```python
from build123d import *

# Parameters (mm, degrees)
SKETCH_1_W          = 206.4
SKETCH_1_H          = 150
SKETCH_1_R          = 2.1
SKETCH_1_R_2        = 1.5
EXTRUDE_1_DEPTH     = 3
CUT_EXTRUDE_1_DEPTH = 153.892903694
FILLET_1_R          = 3
CUT_EXTRUDE_2_DEPTH = 2
SKETCH_6_R          = 10
CUT_EXTRUDE_3_DEPTH = 10
SKETCH_7_W          = 45
SKETCH_7_H          = 100
CUT_EXTRUDE_4_DEPTH = 10
FILLET_2_R          = 3
SKETCH_8_W          = 45.884132908
SKETCH_8_H          = 94.377965814
CUT_EXTRUDE_5_DEPTH = 10
SKETCH_9_W          = 66.4
SKETCH_9_H          = 90
CUT_EXTRUDE_6_DEPTH = 10
SKETCH_10_R         = 1.5
CUT_EXTRUDE_7_DEPTH = 2


with BuildPart() as part:
    # 草图1 → 凸台-拉伸1 (new body)
    with BuildSketch(Plane(origin=(0, 0, 0), x_dir=(1, 0, 0), z_dir=(0, 1, 0))):
        with Locations((-30, 0)):
            Rectangle(SKETCH_1_W, SKETCH_1_H)
        with Locations(Location((65.7, 67.5, 0), (0, 0, 270))):
            Circle(SKETCH_1_R, mode=Mode.SUBTRACT)
        with Locations(Location((65.7, -67.5, 0), (0, 0, 90))):
            Circle(SKETCH_1_R, mode=Mode.SUBTRACT)
        with Locations(Location((-65.7, -67.5, 0), (0, 0, 270))):
            Circle(SKETCH_1_R, mode=Mode.SUBTRACT)
        with Locations(Location((-65.7, 67.5, 0), (0, 0, 90))):
            Circle(SKETCH_1_R, mode=Mode.SUBTRACT)
        with Locations(Location((-65.7, 37.5, 0), (0, 0, 270))):
            Circle(SKETCH_1_R, mode=Mode.SUBTRACT)
        with Locations(Location((-40.7, 37.5, 0), (0, 0, 270))):
            Circle(SKETCH_1_R, mode=Mode.SUBTRACT)
        with Locations(Location((-40.7, 67.5, 0), (0, 0, 270))):
            Circle(SKETCH_1_R, mode=Mode.SUBTRACT)
        with Locations(Location((-40.7, -67.5, 0), (0, 0, 270))):
            Circle(SKETCH_1_R, mode=Mode.SUBTRACT)
        with Locations(Location((-40.7, -37.5, 0), (0, 0, 270))):
            Circle(SKETCH_1_R, mode=Mode.SUBTRACT)
        with Locations(Location((-65.7, -37.5, 0), (0, 0, 270))):
            Circle(SKETCH_1_R, mode=Mode.SUBTRACT)
        with Locations(Location((40.7, -67.5, 0), (0, 0, 270))):
            Circle(SKETCH_1_R, mode=Mode.SUBTRACT)
        with Locations(Location((40.7, -37.5, 0), (0, 0, 270))):
            Circle(SKETCH_1_R, mode=Mode.SUBTRACT)
        with Locations(Location((65.7, -37.5, 0), (0, 0, 270))):
            Circle(SKETCH_1_R, mode=Mode.SUBTRACT)
        with Locations(Location((65.7, 37.5, 0), (0, 0, 270))):
            Circle(SKETCH_1_R, mode=Mode.SUBTRACT)
        with Locations(Location((40.7, 37.5, 0), (0, 0, 270))):
            Circle(SKETCH_1_R, mode=Mode.SUBTRACT)
        with Locations(Location((40.7, 67.5, 0), (0, 0, 270))):
            Circle(SKETCH_1_R, mode=Mode.SUBTRACT)
        with Locations(Location((-98.4, 63.575, 0), (0, 0, 270))):
            Circle(SKETCH_1_R_2, mode=Mode.SUBTRACT)
        with Locations(Location((-88.4, 63.575, 0), (0, 0, 270))):
            Circle(SKETCH_1_R_2, mode=Mode.SUBTRACT)
        with Locations(Location((-111.4, 63.575, 0), (0, 0, 270))):
            Circle(SKETCH_1_R_2, mode=Mode.SUBTRACT)
        with Locations(Location((-121.4, 63.575, 0), (0, 0, 270))):
            Circle(SKETCH_1_R_2, mode=Mode.SUBTRACT)
        with Locations(Location((-121.4, -63.474999999, 0), (0, 0, 270))):
            Circle(SKETCH_1_R_2, mode=Mode.SUBTRACT)
        with Locations(Location((-111.4, -63.474999999, 0), (0, 0, 270))):
            Circle(SKETCH_1_R_2, mode=Mode.SUBTRACT)
        with Locations(Location((-98.4, -63.425, 0), (0, 0, 270))):
            Circle(SKETCH_1_R_2, mode=Mode.SUBTRACT)
        with Locations(Location((-88.4, -63.425, 0), (0, 0, 270))):
            Circle(SKETCH_1_R_2, mode=Mode.SUBTRACT)
    extrude(amount=EXTRUDE_1_DEPTH)

    # 草图2 → 切除-拉伸1 (cut, through all)
    with BuildSketch(Plane(origin=(0, 0, 0), x_dir=(1, 0, 0), z_dir=(0, 1, 0))):
        with BuildLine():
            Line((-125.2, -66.425), (-116.5, -66.425))
            ThreePointArc((-116.5, -66.425), (-114.9, -64.825), (-113.3, -66.425))
            Line((-113.3, -66.425), (-113.3, -69.575))
            ThreePointArc((-113.3, -69.575), (-114.9, -71.175), (-116.5, -69.575))
            Line((-116.5, -69.575), (-125.2, -69.575))
            ThreePointArc((-125.2, -69.575), (-126.8, -71.175), (-128.4, -69.575))
            Line((-128.4, -69.575), (-128.4, -66.425))
            ThreePointArc((-128.4, -66.425), (-126.8, -64.825), (-125.2, -66.425))
        make_face()
        with BuildLine():
            Line((-85.2, -66.425), (-76.5, -66.425))
            ThreePointArc((-76.5, -66.425), (-74.9, -64.825), (-73.3, -66.425))
            Line((-73.3, -66.425), (-73.3, -69.575))
            ThreePointArc((-73.3, -69.575), (-74.9, -71.175), (-76.5, -69.575))
            Line((-76.5, -69.575), (-85.2, -69.575))
            ThreePointArc((-85.2, -69.575), (-86.8, -71.175), (-88.4, -69.575))
            Line((-88.4, -69.575), (-88.4, -66.425))
            ThreePointArc((-88.4, -66.425), (-86.8, -64.825), (-85.2, -66.425))
        make_face()
        with BuildLine():
            Line((-73.3, 66.425), (-73.3, 69.575))
            ThreePointArc((-73.3, 69.575), (-74.9, 71.175), (-76.5, 69.575))
            Line((-76.5, 69.575), (-85.2, 69.575))
            ThreePointArc((-85.2, 69.575), (-86.8, 71.175), (-88.4, 69.575))
            Line((-88.4, 69.575), (-88.4, 66.425))
            ThreePointArc((-88.4, 66.425), (-86.8, 64.825), (-85.2, 66.425))
            Line((-85.2, 66.425), (-76.5, 66.425))
            ThreePointArc((-76.5, 66.425), (-74.9, 64.825), (-73.3, 66.425))
        make_face()
        with BuildLine():
            Line((-113.3, 66.425), (-113.3, 69.575))
            ThreePointArc((-113.3, 69.575), (-114.9, 71.175), (-116.5, 69.575))
            Line((-116.5, 69.575), (-125.2, 69.575))
            ThreePointArc((-125.2, 69.575), (-126.8, 71.175), (-128.4, 69.575))
            Line((-128.4, 69.575), (-128.4, 66.425))
            ThreePointArc((-128.4, 66.425), (-126.8, 64.825), (-125.2, 66.425))
            Line((-125.2, 66.425), (-116.5, 66.425))
            ThreePointArc((-116.5, 66.425), (-114.9, 64.825), (-113.3, 66.425))
        make_face()
    extrude(amount=CUT_EXTRUDE_1_DEPTH, mode=Mode.SUBTRACT)

    # 圆角1
    fillet_1_edges = [part.edges().sort_by_distance(p)[0] for p in [
        (73.2, 1.5, 75),
        (-133.2, 1.5, 75),
        (-133.2, 1.5, -75),
        (73.2, 1.5, -75),
    ]]
    fillet(fillet_1_edges, radius=FILLET_1_R)

    # 草图4 → 切除-拉伸2 (cut)
    with BuildSketch(Plane(origin=(0, 0, 0), x_dir=(1, 0, 0), z_dir=(0, 1, 0))):
        with BuildLine():
            Line((-120.7, -27.5), (60.7, -27.5))
            ThreePointArc((60.7, -27.5), (64.235533906, -26.035533906), (65.7, -22.5))
            Line((65.7, -22.5), (65.7, 22.5))
            ThreePointArc((65.7, 22.5), (64.235533906, 26.035533906), (60.7, 27.5))
            Line((60.7, 27.5), (-120.7, 27.5))
            ThreePointArc((-120.7, 27.5), (-124.235533906, 26.035533906), (-125.7, 22.5))
            Line((-125.7, 22.5), (-125.7, -22.5))
            ThreePointArc((-125.7, -22.5), (-124.235533906, -26.035533906), (-120.7, -27.5))
        make_face()
    extrude(amount=CUT_EXTRUDE_2_DEPTH, mode=Mode.SUBTRACT)

    # 草图6 → 切除-拉伸3 (cut)
    with BuildSketch(Plane(origin=(0, 3, 0), x_dir=(1, 0, 0), z_dir=(0, 1, 0))):
        with Locations(Location((0, 0, 0), (0, 0, 270))):
            Circle(SKETCH_6_R)
    extrude(amount=-CUT_EXTRUDE_3_DEPTH, mode=Mode.SUBTRACT)

    # 草图7 → 切除-拉伸4 (cut)
    with BuildSketch(Plane(origin=(0, 3, 0), x_dir=(1, 0, 0), z_dir=(0, 1, 0))):
        with Locations((-110.7, 0)):
            Rectangle(SKETCH_7_W, SKETCH_7_H)
    extrude(amount=-CUT_EXTRUDE_4_DEPTH, mode=Mode.SUBTRACT)

    # 圆角2
    fillet_2_edges = [part.edges().sort_by_distance(p)[0] for p in [
        (-133.2, 1.5, 50),
        (-133.2, 1.5, -50),
        (-88.2, 1.5, -50),
        (-88.2, 1.5, 50),
    ]]
    fillet(fillet_2_edges, radius=FILLET_2_R)

    # 草图8 → 切除-拉伸5 (cut)
    with BuildSketch(Plane(origin=(0, 3, 0), x_dir=(1, 0, 0), z_dir=(0, 1, 0))):
        Rectangle(SKETCH_8_W, SKETCH_8_H)
    extrude(amount=-CUT_EXTRUDE_5_DEPTH, mode=Mode.SUBTRACT)

    # 草图9 → 切除-拉伸6 (cut)
    with BuildSketch(Plane(origin=(0, 3, 0), x_dir=(1, 0, 0), z_dir=(0, 1, 0))):
        with Locations((-1e-09, 0)):
            Rectangle(SKETCH_9_W, SKETCH_9_H)
    extrude(amount=-CUT_EXTRUDE_6_DEPTH, mode=Mode.SUBTRACT)

    # 草图10 → 切除-拉伸7 (cut)
    with BuildSketch(Plane(origin=(0, 3, 0), x_dir=(1, 0, 0), z_dir=(0, 1, 0))):
        with Locations(Location((-15, 60.780217665, 0), (0, 0, 270))):
            Circle(SKETCH_10_R)
        with Locations(Location((15, 60.780217665, 0), (0, 0, 90))):
            Circle(SKETCH_10_R)
        with Locations(Location((15, -60.780217665, 0), (0, 0, 270))):
            Circle(SKETCH_10_R)
        with Locations(Location((-15, -60.780217665, 0), (0, 0, 90))):
            Circle(SKETCH_10_R)
    extrude(amount=-CUT_EXTRUDE_7_DEPTH, mode=Mode.SUBTRACT)


solid = part.part
```
Model file for the job. Use its own axes, mm. A direction names the side the tool comes from. Give positions to 0.01 mm unless a question says otherwise; leave off trailing zeros. Loops run counter-clockwise (first coordinate to the right, second up) from the corner with the lowest first, then second, coordinate; pieces in that order, holes last. Notation, with made-up numbers: (73.25, 69.5) - (91.25, 69.5) arc R28 ccw to (91.25, 89.5) - close; hole circle Ø5 at (62, -14.75). An arc over 180 degrees is marked (long way). One line per item, written item: value. Start each with the question number.
1. Probe L1, parallel to X at y = 2, z = 37.5; L2, parallel to X at y = 0.6, z = -63.5; L3, parallel to Z at x = -41, y = 0.9. List the from-to ranges inside material, lowest first. Write a range as from..to.
2. Slice it at C-C (z = -37.5). List the corners of the cut face in (x, y).
3. Slice it at A-A (x = 40.7). List the corners of the cut face in (y, z), plus the area to 3 significant figures.
4. Pin check, flat tips, straight feed: pin 1 (0.9 mm diameter, centred on x = -15.5, z = 61.5, fed in from +Y); pin 2 (16.5 mm diameter, centred on x = -51, z = 11, fed in from -Y). Stop position of each tip, or through.
5. Pull direction X, two halves, no side cores. Call faces 3 (the cylindrical face through (39.422, 1.479, -39.166)), 4 (the cylindrical face through (64.2, 0.99, 26.07)), 5 (the cylindrical face through (63.65, 1.48, -67.96)), 6 (the flat face through (-54, 3, -1)): pulls with the +X half, pulls with the -X half, needs draft (parallel to the pull), parting line crosses it, or undercut.
6. Which spindle directions (+Z, -Z, +X, -X, +Y, -Y) get a long thin tool onto all of the face, cutting with end or side? Do faces 1 (the cylindrical face through (63.65, 1.48, -37.96)), 2 (the flat face through (49, 2, 0)). Say none if no direction does.
7. Slice it at D-D (x = -8). List the corners of the cut face in (y, z), plus the area to 3 significant figures.
8. Slice it at B-B (x = -81). List the corners of the cut face in (y, z) (3 decimals).
Solution:
1. L1: x = -88.2..-67.8, -63.6..-42.8, -38.6..-33.2, 33.2..38.6, 42.8..63.6, 67.8..73.2
1. L2: x = -133.2..-122.9, -119.9..-112.9, -109.9..-99.9, -96.9..-89.9, -86.9..73.2
1. L3: z = -75..-69.58, -65.42..-39.58, -35.42..-27.5, 27.5..35.42, 39.58..65.42, 69.58..75
2. outline: (-88.2, 0) - (-67.8, 0) - (-67.8, 3) - (-88.2, 3) - close; (-63.6, 0) - (-42.8, 0) - (-42.8, 3) - (-63.6, 3) - close; (-38.6, 0) - (-33.2, 0) - (-33.2, 3) - (-38.6, 3) - close; (33.2, 0) - (38.6, 0) - (38.6, 3) - (33.2, 3) - close; (42.8, 0) - (63.6, 0) - (63.6, 3) - (42.8, 3) - close; (67.8, 0) - (73.2, 0) - (73.2, 3) - (67.8, 3) - close
3. outline: (0, -75) - (3, -75) - (3, -69.6) - (0, -69.6) - close; (0, -65.4) - (3, -65.4) - (3, -39.6) - (0, -39.6) - close; (0, -35.4) - (3, -35.4) - (3, 35.4) - (0, 35.4) - (0, 27.5) - (2, 27.5) - (2, -27.5) - (0, -27.5) - close; (0, 39.6) - (3, 39.6) - (3, 65.4) - (0, 65.4) - close; (0, 69.6) - (3, 69.6) - (3, 75) - (0, 75) - close
3. area: 290 mm^2
4. pin 1: stops at y = 1
4. pin 2: stops at y = 2
5. face 3: undercut
5. face 4: pulls with the -X half
5. face 5: undercut
5. face 6: needs draft
6. face 1: +Y, -Y
6. face 2: -X, -Y
7. outline: (0, -75) - (3, -75) - (3, -47.19) - (0, -47.19) - close; (0, 47.19) - (3, 47.19) - (3, 75) - (0, 75) - close
7. area: 167 mm^2
8. outline: (0, -75) - (3, -75) - (3, -69.575) - (0, -69.575) - close; (0, -66.425) - (3, -66.425) - (3, 66.425) - (0, 66.425) - (0, 27.5) - (2, 27.5) - (2, -27.5) - (0, -27.5) - close; (0, 69.575) - (3, 69.575) - (3, 75) - (0, 75) - close
